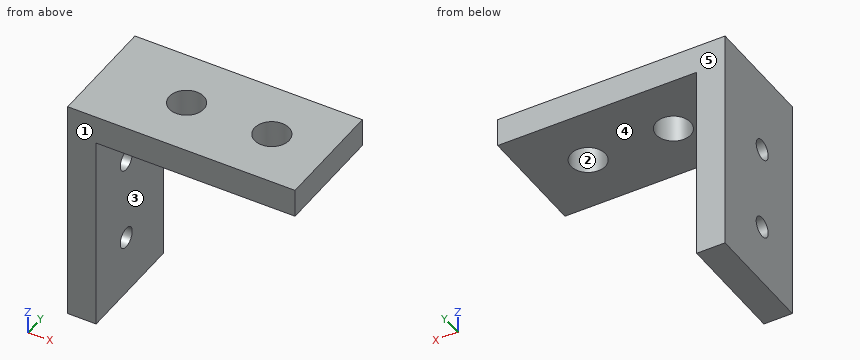
```python
from build123d import *

# Parameters (mm, degrees)
BOSS_EXTRUDE1_DEPTH         = 12.7
F_24_0_152_DIAMETER_HOLE1_D = 3.8608
TAP_DRILL_FOR_4_40_TAP1_D   = 2.2606


with BuildPart() as part:
    # Sketch1 → Boss-Extrude1 (new body)
    with BuildSketch(Plane(origin=(0, 0, 0), x_dir=(1, 0, 0), z_dir=(0, 1, 0))):
        Polygon((-9.525, 12.7), (-9.525, -9.525), (12.7, -9.525), (12.7, -12.7), (-12.7, -12.7), (-12.7, 12.7), align=None)
    extrude(amount=BOSS_EXTRUDE1_DEPTH)

    # #24 (0.152) Diameter Hole1 (through all)
    with Locations(Plane(origin=(6.35, 6.35, 9.525), x_dir=(-1, 0, 0), z_dir=(0, 0, -1))):
        with Locations((0, 0), (9.525, 0)):
            Hole(F_24_0_152_DIAMETER_HOLE1_D / 2)

    # Tap Drill for #4-40 Tap1 (through all)
    with Locations(Plane(origin=(-12.7, 5.6896, -5.969), x_dir=(0, 0, -1), z_dir=(-1, 0, 0))):
        with Locations((0, 0), (-9.4996, 0)):
            Hole(TAP_DRILL_FOR_4_40_TAP1_D / 2)


solid = part.part
```
Check sheet for the modelled part. Datum: model origin and axes. Units: mm. Face numbers are marked on the shaded views. A direction names the side the tool comes from. Give positions to 0.01 mm unless a question says otherwise; leave off trailing zeros. Loops run counter-clockwise (first coordinate to the right, second up) from the corner with the lowest first, then second, coordinate; pieces in that order, holes last. Notation, with made-up numbers: M 56,39 L 97,39 A9 ccw 97,54 Z; hole C 36,25.5 d7. An arc over 180 degrees is marked long. Answer in a Markdown table with one row per item.
1) Depth check by flat-ended pin: pin 1 (4 mm diameter, centred on y = 4, z = 4, fed in from +X) (3 decimals); pin 2 (4 mm diameter, centred on x = -3.5, y = 9.5, fed in from -Z) (3 decimals). Enter the tip coordinate at first touch or a pass-through.
Solutions:
| item | result |
|---|---|
| pin 1 | stops at x = -9.525 |
| pin 2 | stops at z = 9.525 |
2) Cross-section at D-D (x = -2.25). Enter the section's corners in (y, z) (3 decimals).
Solutions:
| item | result |
|---|---|
| outline | M 0,9.525 L 4.656,9.525 L 4.656,12.7 L 0,12.7 Z; M 8.044,9.525 L 12.7,9.525 L 12.7,12.7 L 8.044,12.7 Z |
3) Tool access check on the marked faces 4 and 5. Record the directions out of +Z, -Z, +X, -X, +Y, -Y that give a thin tool (end or side, any length) a straight path to the whole face; none if there is none.
Solutions:
| item | result |
|---|---|
| face 4 | -Z, +X, +Y, -Y |
| face 5 | +Z, -Z, +X, -X, +Y |
4) Mould release check, pull along Y, two halves, no side actions. Record for the marked faces 1, 2 and 3: released by +Y, released by -Y, zero draft, split by the parting line, or undercut.
Solutions:
| item | result |
|---|---|
| face 1 | released by -Y |
| face 2 | undercut |
| face 3 | zero draft |
5) Cross-section at A-A (x = 6.35). Enter the section's corners in (y, z) (3 decimals), plus the area to 3 significant figures.
Solutions:
| item | result |
|---|---|
| outline | M 0,9.525 L 4.42,9.525 L 4.42,12.7 L 0,12.7 Z; M 8.28,9.525 L 12.7,9.525 L 12.7,12.7 L 8.28,12.7 Z |
| area | 28.1 mm^2 |
6) Cross-section at C-C (z = 1.5). Enter the section's corners in (x, y) (3 decimals).
Solutions:
| item | result |
|---|---|
| outline | M -12.7,0 L -9.525,0 L -9.525,12.7 L -12.7,12.7 Z |
7) Cross-section at B-B (y = 7.5). Enter the section's corners in (x, z) (3 decimals), plus the area to 3 significant figures.
Solutions:
| item | result |
|---|---|
| outline | M -12.7,-12.7 L -9.525,-12.7 L -9.525,9.525 L -4.725,9.525 L -4.725,12.7 L -12.7,12.7 Z; M -1.625,9.525 L 4.8,9.525 L 4.8,12.7 L -1.625,12.7 Z; M 7.9,9.525 L 12.7,9.525 L 12.7,12.7 L 7.9,12.7 Z |
| area | 132 mm^2 |
8) Thickness scan on line 1 (X direction, y = 10.75, z = -7.75) (3 decimals); line 2 (Z direction, x = 6.25, y = 10) (3 decimals); line 3 (Y direction, x = 6.35, z = 11.05). Record the ranges inside material, lowest first.
Solutions:
| item | result |
|---|---|
| line 1 | x = -12.7 to -9.525 |
| line 2 | z = 9.525 to 12.7 |
| line 3 | y = 0 to 4.42, 8.28 to 12.7 |
